Geometry: final body of the model. Coordinates: model frame, mm. Face numbers are marked on the shaded views. A direction names the side the tool comes from. Give positions to 0.01 mm unless a question says otherwise; leave off trailing zeros. Loops run counter-clockwise (first coordinate to the right, second up) from the corner with the lowest first, then second, coordinate; pieces in that order, holes last. Notation, with made-up numbers: (9.25, 25) -> (20.25, 25) arc R22 cw to (20.25, 31) -> close; hole circle Ø9 at (33, -19). An arc over 180 degrees is marked (long way). Answer in a Markdown table with one row per item. Add a question column.
1) Line query: line 1 (Z direction, x = -7.5, y = 16); line 2 (X direction, y = 8, z = 8); line 3 (Y direction, x = 13, z = 9). Output: solid intervals per line, ascending. Write a range as from..to.
2) Section query C-C (x = -11.5). Return the cut outline in (y, z), plus the area to 4 significant figures.
3) First-contact query: P1, Ø5, axis at y = -4, z = 18, coming from the +X side; P2, Ø15.5, axis at x = 2.5, z = 21, coming from the +Y side; P3, Ø8, axis at x = -8, y = 2, coming from the +Z side. Flat tips, straight axial feed; report the tip coordinate or a pass-through.
4) Draft query along Y for the marked faces 1, 2, 3 and 4. Return one class per face: +Y half, -Y half, draft (parallel to the pull), parting line (faces both ways), or undercut.
5) Access query for the marked faces 5, 6 and 7. Directions: +Z, -Z, +X, -X, +Y, -Y. A direction counts if a zero-diameter tool reaches every point of the face in a straight line with its end or side. Return the directions, or none.
6) Section query D-D (y = 13.5). Return the cut outline in (x, z).
7) Section query A-A (z = 17.5). Return the cut outline in (x, y).
8) Section query B-B (x = 2.5). Return the cut outline in (y, z), plus the area to 3 significant figures.
```python
from build123d import *

# Parameters (mm, degrees)
F0_W     = 36
F0_H     = 38
F1_DEPTH = 36
F3_DEPTH = 38.001
F4_DEPTH = 33
F6_DEPTH = 36.001


with BuildPart() as f1:
    # F0 (on Top) → F1 (new body)
    with BuildSketch(Plane.XY):
        Rectangle(F0_W, F0_H)
        with BuildLine():
            ThreePointArc((-8.5, 2.35), (-7.914214, 3.764214), (-6.5, 4.35))
            Line((-6.5, 4.35), (9.5, 4.35))
            ThreePointArc((9.5, 4.35), (10.914214, 3.764214), (11.5, 2.35))
            Line((11.5, 2.35), (11.5, -2.35))
            ThreePointArc((11.5, -2.35), (10.914214, -3.764214), (9.5, -4.35))
            Line((9.5, -4.35), (-6.5, -4.35))
            ThreePointArc((-6.5, -4.35), (-7.914214, -3.764214), (-8.5, -2.35))
            Line((-8.5, -2.35), (-8.5, 2.35))
        make_face(mode=Mode.SUBTRACT)
    extrude(amount=F1_DEPTH)

    # F2 (on face) → F3 (cut, through all)
    with BuildSketch(Plane(origin=(0, 19, 0), x_dir=(-1, 0, 0), z_dir=(0, 1, 0))):
        Polygon((-18, 5.5), (12.5, 36), (-18, 36), align=None)
    extrude(amount=-F3_DEPTH, mode=Mode.SUBTRACT)

    # F2 (on face) → F4 (cut)
    with BuildSketch(Plane(origin=(0, 19, 0), x_dir=(-1, 0, 0), z_dir=(0, 1, 0))):
        Polygon((12.5, 5.5), (12.5, 36), (-18, 5.5), align=None)
    extrude(amount=-F4_DEPTH, mode=Mode.SUBTRACT)

    # F5 (on face) → F6 (cut, through all)
    with BuildSketch(Plane(origin=(-18, 0, 0), x_dir=(0, -1, 0), z_dir=(-1, 0, 0))):
        with BuildLine():
            Line((2.35, 29.5), (-2.35, 29.5))
            ThreePointArc((-2.35, 29.5), (-3.764214, 28.914214), (-4.35, 27.5))
            Line((-4.35, 27.5), (-4.35, 11.5))
            ThreePointArc((-4.35, 11.5), (-3.764214, 10.085786), (-2.35, 9.5))
            Line((-2.35, 9.5), (2.35, 9.5))
            ThreePointArc((2.35, 9.5), (3.764214, 10.085786), (4.35, 11.5))
            Line((4.35, 11.5), (4.35, 27.5))
            ThreePointArc((4.35, 27.5), (3.764214, 28.914214), (2.35, 29.5))
        make_face()
    extrude(amount=-F6_DEPTH, mode=Mode.SUBTRACT)


solid = f1.part
```
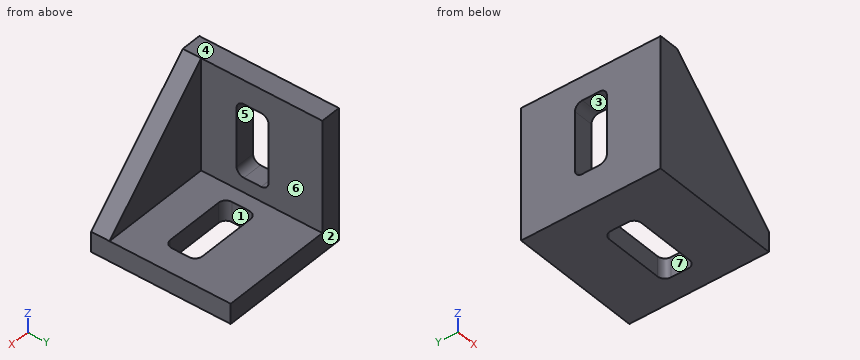
Evaluation:
| question | item | result |
|---|---|---|
| 1 | line 1 | 0..5.5 |
| 1 | line 2 | -18..-12.5 |
| 1 | line 3 | -19..-14 |
| 2 | outline | (-19, 0) -> (19, 0) -> (19, 5.5) -> (-14, 5.5) -> (-14, 35) -> (-19, 35) -> close |
| 2 | area | 356.5 mm² |
| 3 | P1 | x = -12.5 |
| 3 | P2 | y = -14 |
| 3 | P3 | z = 5.5 |
| 4 | face 1 | undercut |
| 4 | face 2 | +Y half |
| 4 | face 3 | undercut |
| 4 | face 4 | draft |
| 5 | face 5 | +X, -X |
| 5 | face 6 | +Z, +X, +Y |
| 5 | face 7 | +Z, -Z |
| 6 | outline | (-18, 0) -> (18, 0) -> (18, 5.5) -> (-12.5, 5.5) -> (-12.5, 36) -> (-18, 36) -> close |
| 7 | outline | (-18, -19) -> (6, -19) -> (6, -14) -> (-12.5, -14) -> (-12.5, -4.35) -> (-18, -4.35) -> close; (-18, 4.35) -> (-12.5, 4.35) -> (-12.5, 19) -> (-18, 19) -> close |
| 8 | outline | (-19, 0) -> (-4.35, 0) -> (-4.35, 5.5) -> (-14, 5.5) -> (-14, 21) -> (-19, 21) -> close; (4.35, 0) -> (19, 0) -> (19, 5.5) -> (4.35, 5.5) -> close |
| 8 | area | 239 mm² |
